from build123d import *

# Parameters (mm, degrees)
SKIZZE1_W                       = 49.2
SKIZZE1_H                       = 24.6
AUFSATZ_LINEAR_AUSTRAGEN1_DEPTH = 1
AUFSATZ_LINEAR_AUSTRAGEN2_DEPTH = 1.4
AUFSATZ_LINEAR_AUSTRAGEN3_DEPTH = 1
AUFSATZ_LINEAR_AUSTRAGEN4_DEPTH = 0.5
SKIZZE6_W                       = 4
SKIZZE6_H                       = 5
AUFSATZ_LINEAR_AUSTRAGEN5_DEPTH = 6
SKIZZE7_R                       = 1.3
SCHNITT_LINEAR_AUSTRAGEN1_DEPTH = 4
VERRUNDUNG1_R                   = 1
SCHNITT_LINEAR_AUSTRAGEN2_DEPTH = 1


with BuildPart() as part:
    # Skizze1 → Aufsatz-Linear austragen1 (new body)
    with BuildSketch(Plane(origin=(0, 0, 0), x_dir=(1, 0, 0), z_dir=(0, 1, 0))):
        Rectangle(SKIZZE1_W, SKIZZE1_H)
    extrude(amount=AUFSATZ_LINEAR_AUSTRAGEN1_DEPTH)

    # Skizze2 → Aufsatz-Linear austragen2 (add)
    with BuildSketch(Plane.XY.offset(12.3)):
        Polygon((17.9, 0), (-17.9, 0), (-6.35, 19.8), (6.35, 19.8), align=None)
    extrude(amount=AUFSATZ_LINEAR_AUSTRAGEN2_DEPTH)

    # Skizze4 → Aufsatz-Linear austragen3 (add)
    with BuildSketch(Plane(origin=(0, 0, 12.3), x_dir=(-1, 0, 0), z_dir=(0, 0, -1))):
        Polygon((6.35, 20.9), (17.958333333, 1), (-17.958333333, 1), (-6.35, 20.9), align=None)
    extrude(amount=AUFSATZ_LINEAR_AUSTRAGEN3_DEPTH)

    # Skizze5 → Aufsatz-Linear austragen4 (add, symmetric)
    with BuildSketch(Plane(origin=(5, 0, 0), x_dir=(0, 0, -1), z_dir=(1, 0, 0))):
        Polygon((-6.3, 1), (-11.3, 15.9), (-11.3, 1), align=None)
    aufsatz_linear_austragen4 = extrude(amount=AUFSATZ_LINEAR_AUSTRAGEN4_DEPTH, both=True)

    # Spiegeln1: Aufsatz-Linear austragen4 across plane
    add(aufsatz_linear_austragen4.mirror(Plane(origin=(0, 0, 0), x_dir=(0, 0, 1), z_dir=(1, 0, 0))))

    # Skizze6 → Aufsatz-Linear austragen5 (add)
    with BuildSketch(Plane(origin=(0, 1, 0), x_dir=(1, 0, 0), z_dir=(0, 1, 0))):
        with Locations((-21.5, 0)):
            Rectangle(SKIZZE6_W, SKIZZE6_H)
    aufsatz_linear_austragen5 = extrude(amount=AUFSATZ_LINEAR_AUSTRAGEN5_DEPTH)

    # Skizze7 → Schnitt-Linear austragen1 (cut)
    with BuildSketch(Plane.ZY.offset(23.5)):
        with Locations((0, 4)):
            Circle(SKIZZE7_R)
    schnitt_linear_austragen1 = extrude(amount=-SCHNITT_LINEAR_AUSTRAGEN1_DEPTH, mode=Mode.SUBTRACT)

    # Spiegeln2: Aufsatz-Linear austragen5, Schnitt-Linear austragen1 across plane
    add(aufsatz_linear_austragen5.mirror(Plane(origin=(0, 0, 0), x_dir=(0, 0, 1), z_dir=(1, 0, 0))))
    add(schnitt_linear_austragen1.mirror(Plane(origin=(0, 0, 0), x_dir=(0, 0, 1), z_dir=(1, 0, 0))), mode=Mode.SUBTRACT)

    # Verrundung1
    verrundung1_edges = [part.edges().sort_by_distance(p)[0] for p in [
        (0, 0, 13.7),
    ]]
    fillet(verrundung1_edges, radius=VERRUNDUNG1_R)

    # Skizze8 → Schnitt-Linear austragen2 (cut)
    with BuildSketch(Plane.XZ):
        with BuildLine():
            Line((3.3, -5.4), (-3.3, -5.4))
            ThreePointArc((-3.3, -5.4), (-4.148528137, -5.751471863), (-4.5, -6.6))
            Line((-4.5, -6.6), (-4.5, -7.4))
            ThreePointArc((-4.5, -7.4), (-4.148528137, -8.248528137), (-3.3, -8.6))
            Line((-3.3, -8.6), (3.3, -8.6))
            ThreePointArc((3.3, -8.6), (4.148528137, -8.248528137), (4.5, -7.4))
            Line((4.5, -7.4), (4.5, -6.6))
            ThreePointArc((4.5, -6.6), (4.148528137, -5.751471863), (3.3, -5.4))
        make_face()
    extrude(amount=-SCHNITT_LINEAR_AUSTRAGEN2_DEPTH, mode=Mode.SUBTRACT)


solid = part.part
Design review of the part built by this model. Coordinates are the model's own, in mm. A direction names the side the tool comes from. Round coordinates to 2 decimals unless told otherwise and drop trailing zeros. Write each loop counter-clockwise with the first axis right and the second up, starting at its lowest first coordinate (ties: lowest second). Pieces come first, ordered by that corner, then holes. Notation, with made-up numbers: (-19, -35) - (4, -35) arc R35 cw to (4, 0) - close; hole circle Ø7 at (-11, -4). An arc over 180 degrees is marked (long way). Use a Markdown table: item, result. Add a question column.
1. Wall thickness on probe 1 along Y at (x, z) = (21.2, 0); probe 2 along X at (y, z) = (9.25, 9.25); probe 3 along Y at (x, z) = (-12.5, 8.5): over which ranges is each line inside the solid? List them lowest first.
2. We need section B-B (y = 4). Count the separate pieces of the cut face and the enclosed holes in it, then the cut area to 3 significant figures.
3. Mouldability with a two-part tool opening along Y and no side actions: class faces 1 (the face through (-21.53, 2.73, -0.28)), 2 (the face through (-19.5, 2.6, 0.6)), 3 (the face through (21.53, 2.73, -0.28)), 4 (the face through (-12.073, 11.089, 11.807)) as +Y half, -Y half, draft (parallel to the pull), parting line (faces both ways), or undercut.
4. Clearance check with flat-ended pins moving along their axes: pin 1 (3 mm diameter, centred on y = 8, z = 9.5, fed in from -X); pin 2 (3 mm diameter, centred on x = -21.5, y = 4.5, fed in from -Z); pin 3 (5 mm diameter, centred on x = -7, z = 4.5, fed in from -Y); pin 4 (2.5 mm diameter, centred on y = 4.5, z = -1, fed in from -X). State where each tip first meets the part, or that it passes through.
5. For faces 5 (the face through (22, 4, -2.5)), 6 (the face through (12.044, 10.039, 12.99)), 7 (the face through (0, 0.5, -5.4)), 8 (the face through (22, 4, 2.5)), list the 3-axis set-ups (+Z, -Z, +X, -X, +Y, -Y) from which the entire face can be reached by the end or side of a thin tool; tool diameter is ignored.
6. We need section C-C (x = -12). State the section outline as (y, z) points.
7. We need section A-A (z = 0). State the section outline as (x, y) points, then the cut area to 3 significant figures.
8. We need section D-D (y = 13.75). State the section outline as (x, z) points, then the cut area to 3 significant figures.
Output:
| question | item | result |
|---|---|---|
| 1 | probe 1 | y = 0 to 2.7, 5.3 to 7 |
| 1 | probe 2 | x = -5.5 to -4.5, 4.5 to 5.5 |
| 1 | probe 3 | y = 0 to 1 |
| 2 | separate pieces | 5 |
| 2 | enclosed holes | 0 |
| 2 | area | 103 mm2 |
| 3 | face 1 | undercut |
| 3 | face 2 | draft |
| 3 | face 3 | undercut |
| 3 | face 4 | +Y half |
| 4 | pin 1 | stops at x = -5.5 |
| 4 | pin 2 | stops at z = -2.5 |
| 4 | pin 3 | stops at y = 0 |
| 4 | pin 4 | stops at x = -23.5 |
| 5 | face 5 | -Z, +X, -X, +Y |
| 5 | face 6 | +Z, +X, +Y |
| 5 | face 7 | +Y, -Y |
| 5 | face 8 | +Z, +X, -X, +Y |
| 6 | outline | (0, -12.3) - (1, -12.3) - (1, 11.3) - (11.21, 11.3) - (11.21, 12.3) - (10.11, 12.3) - (10.11, 13.7) - (1, 13.7) arc R1 ccw to (0, 12.7) - close |
| 7 | outline | (-24.6, 0) - (24.6, 0) - (24.6, 1) - (23.5, 1) - (23.5, 2.7) - (19.5, 2.7) - (19.5, 1) - (-19.5, 1) - (-19.5, 2.7) - (-23.5, 2.7) - (-23.5, 1) - (-24.6, 1) - close; (-23.5, 5.3) - (-19.5, 5.3) - (-19.5, 7) - (-23.5, 7) - close; (19.5, 5.3) - (23.5, 5.3) - (23.5, 7) - (19.5, 7) - close |
| 7 | area | 76.4 mm2 |
| 8 | outline | (-10.52, 11.3) - (-5.5, 11.3) - (-5.5, 10.58) - (-4.5, 10.58) - (-4.5, 11.3) - (4.5, 11.3) - (4.5, 10.58) - (5.5, 10.58) - (5.5, 11.3) - (10.52, 11.3) - (10.52, 12.3) - (9.88, 12.3) - (9.88, 13.7) - (-9.88, 13.7) - (-9.88, 12.3) - (-10.52, 12.3) - close |
| 8 | area | 50.1 mm2 |
